from build123d import *

# Parameters (mm, degrees)
F0_W     = 20.32
F0_H     = 40.64
F1_DEPTH = 35.56
F3_DEPTH = 3.175
F4_R     = 3.175
F5_DEPTH = 3.175
F6_R     = 9.525
F7_DEPTH = 1.5875


with BuildPart() as f1:
    # F0 (on Top) → F1 (new body)
    with BuildSketch(Plane.XY):
        Rectangle(F0_W, F0_H)
    extrude(amount=F1_DEPTH)

    # F2 (on face) → F3 (join)
    with BuildSketch(Plane.XY.offset(35.56)):
        with BuildLine():
            Line((-10.16, 26.67), (-10.16, 20.32))
            Line((-10.16, 20.32), (10.16, 20.32))
            Line((10.16, 20.32), (10.16, 26.67))
            Line((10.16, 26.67), (6.50875, 26.67))
            ThreePointArc((6.50875, 26.67), (6.862802, 25.994267), (6.985, 25.24125))
            ThreePointArc((6.985, 25.24125), (3.850733, 22.982198), (2.69875, 26.67))
            Line((2.69875, 26.67), (-2.69875, 26.67))
            ThreePointArc((-2.69875, 26.67), (-2.344698, 25.994267), (-2.2225, 25.24125))
            ThreePointArc((-2.2225, 25.24125), (-5.356767, 22.982198), (-6.50875, 26.67))
            Line((-6.50875, 26.67), (-10.16, 26.67))
        make_face()
        with BuildLine():
            Line((10.16, -20.32), (-10.16, -20.32))
            Line((-10.16, -20.32), (-10.16, -26.67))
            Line((-10.16, -26.67), (-6.50875, -26.67))
            ThreePointArc((-6.50875, -26.67), (-5.356767, -22.982198), (-2.2225, -25.24125))
            ThreePointArc((-2.2225, -25.24125), (-2.344698, -25.994267), (-2.69875, -26.67))
            Line((-2.69875, -26.67), (2.69875, -26.67))
            ThreePointArc((2.69875, -26.67), (3.850733, -22.982198), (6.985, -25.24125))
            ThreePointArc((6.985, -25.24125), (6.862802, -25.994267), (6.50875, -26.67))
            Line((6.50875, -26.67), (10.16, -26.67))
            Line((10.16, -26.67), (10.16, -20.32))
        make_face()
    extrude(amount=-F3_DEPTH)

    # F4 (on face) → F5 (join)
    with BuildSketch(Plane.XY.offset(35.56)):
        with Locations((0, 13.97)):
            Circle(F4_R)
    extrude(amount=F5_DEPTH)

    # F6 (on face) → F7 (join)
    with BuildSketch(Plane.XY.offset(38.735)):
        with Locations((0, 13.97)):
            Circle(F6_R)
    extrude(amount=F7_DEPTH)


solid = f1.part
Part model, mm, in its own coordinate system. A direction names the side the tool comes from. Coordinates: 2 decimals unless noted, no trailing zeros. Loops run counter-clockwise (first coordinate to the right, second up) from the corner with the lowest first, then second, coordinate; pieces in that order, holes last. Notation, with made-up numbers: (32.5, 66) - (90.5, 66) arc R25 cw to (90.5, 105) - close; hole circle Ø9 at (-28, -7). An arc over 180 degrees is marked (long way). Write each question's results on one line, items separated by ' | '. Start each with the question number.
Q1. Drop flat-ended pins along their axis: pin 1 Ø1.5 at (x, z) = (7, 21) entering from +Y; pin 2 Ø5 at (x, y) = (-1.5, 23) entering from -Z (3 decimals); pin 3 Ø6 at (x, y) = (-4.6, -25.24) entering from +Z. Give the stop position or say it passes through.
Q2. Probe line 1 along Z through (x, y) = (-1, 5.5) (1 decimal); line 2 along Y through (x, z) = (-1.25, 22.5); line 3 along Z through (x, y) = (-0.5, -13). List the from-to ranges inside material, lowest first.
Q3. Which spindle directions (+Z, -Z, +X, -X, +Y, -Y) get a long thin tool onto all of the face, cutting with end or side? Do faces 1 (the flat face through (0, 20.32, 16)), 2 (the cylindrical face through (-0.69, 10.87, 37.13)), 3 (the flat face through (0, -20.32, 16)), 4 (the cylindrical face through (-2.06, 4.67, 39.52)), 5 (the flat face through (8, -26.67, 34)). Say none if no direction does.
Q4. Slice it at D-D on z = 24.5. Give the cut face in (x, y), and give its area (3 significant figures).
Q5. Slice it at B-B on y = 13.97. Give the cut face in (x, z) (1 decimal).
Q6. Slice it at A-A on x = 0. Give the cut face in (y, z) (1 decimal).
Q7. Two-plate mould, pull along Z, no slides. Class faces 6 (the flat face through (0, -23, 32.385)), 7 (the flat face through (0, 10, 38.735)), 8 (the flat face through (0, 14, 40.322)), 9 (the flat face through (8, 26.67, 34)): +Z half, -Z half, draft (parallel to the pull), parting line (faces both ways), or undercut.
Q8. Slice it at C-C on x = 5.5. Give the cut face in (y, z) (1 decimal).
Answer:
1) pin 1: stops at y = 20.32 | pin 2: stops at z = 32.385 | pin 3: stops at z = 35.56
2) line 1: z = 0 to 35.6, 38.7 to 40.3 | line 2: y = -20.32 to 20.32 | line 3: z = 0 to 35.56
3) face 1: -Z, +X, -X, +Y | face 2: none | face 3: -Z, +X, -X, -Y | face 4: +Z | face 5: +Z, -Z, +X, -X, -Y
4) outline: (-10.16, -20.32) - (10.16, -20.32) - (10.16, 20.32) - (-10.16, 20.32) - close | area: 826 mm2
5) outline: (-10.2, 0) - (10.2, 0) - (10.2, 35.6) - (3.2, 35.6) - (3.2, 38.7) - (9.5, 38.7) - (9.5, 40.3) - (-9.5, 40.3) - (-9.5, 38.7) - (-3.2, 38.7) - (-3.2, 35.6) - (-10.2, 35.6) - close
6) outline: (-26.7, 32.4) - (-20.3, 32.4) - (-20.3, 0) - (20.3, 0) - (20.3, 32.4) - (26.7, 32.4) - (26.7, 35.6) - (17.1, 35.6) - (17.1, 38.7) - (23.5, 38.7) - (23.5, 40.3) - (4.4, 40.3) - (4.4, 38.7) - (10.8, 38.7) - (10.8, 35.6) - (-26.7, 35.6) - close
7) face 6: -Z half | face 7: undercut | face 8: +Z half | face 9: draft
8) outline: (-23, 32.4) - (-20.3, 32.4) - (-20.3, 0) - (20.3, 0) - (20.3, 32.4) - (23, 32.4) - (23, 35.6) - (-23, 35.6) - close; (6.2, 38.7) - (21.7, 38.7) - (21.7, 40.3) - (6.2, 40.3) - close
